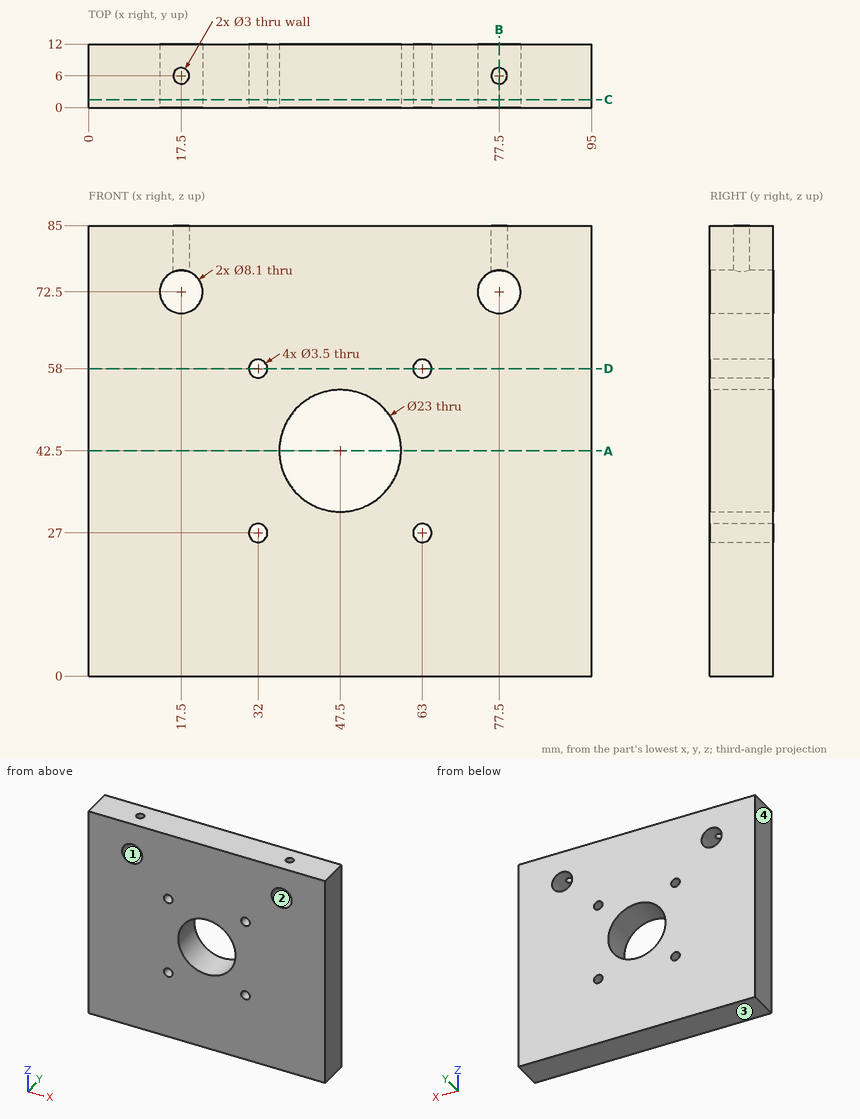
The drawing under review shows one solid part. Ordinate dimensions are in mm from its lowest x, y, z. Coordinates: 2 decimals unless noted, no trailing zeros. Write each loop counter-clockwise with the first axis right and the second up, starting at its lowest first coordinate (ties: lowest second). Pieces come first, ordered by that corner, then holes. Notation, with made-up numbers: (81.5, -1) -> (89.5, -1) arc R20 cw to (89.5, 14) -> close; hole circle Ø2 at (67, -26.75). An arc over 180 degrees is marked (long way). One line per item, written item: value. Start each with the question number.
Q1. Clearance check with a flat-ended pin moving along its axis: P1, Ø14, axis at x = 47.5, z = 42.5, coming from the +Y side. State where the tip first meets the part, or that it passes through.
Q2. Add section A-A, the plane z = 42.5. Give the boundary of the cut face in (x, y), then the cut area to 3 significant figures.
Q3. Add section D-D, the plane z = 58. Give the boundary of the cut face in (x, y).
Q4. Add section B-B, the plane x = 77.5. Give the boundary of the cut face in (y, z), then the cut area to 3 significant figures.
Q5. To check wall thickness, follow probe 1 along X at (y, z) = (6, 27); probe 2 along X at (y, z) = (7.5, 72.5); probe 3 along Z at (x, y) = (64, 7.5). State the ranges of each line that lie inside material, in increasing order.
Q6. Add section C-C, the plane y = 1.5. Give the boundary of the cut face in (x, z), then the cut area to 3 significant figures.
Q7. The part is to be moulded in two halves that separate along X. For the marked faces 1, 2, 3 and 4, say which applies: +X half, -X half, draft (parallel to the pull), parting line (faces both ways), or undercut.
Response:
1. P1: through
2. outline: (0, 0) -> (36, 0) -> (36, 12) -> (0, 12) -> close; (59, 0) -> (95, 0) -> (95, 12) -> (59, 12) -> close
2. area: 864 mm²
3. outline: (0, 0) -> (30.25, 0) -> (30.25, 12) -> (0, 12) -> close; (33.75, 0) -> (61.25, 0) -> (61.25, 12) -> (33.75, 12) -> close; (64.75, 0) -> (95, 0) -> (95, 12) -> (64.75, 12) -> close
4. outline: (0, 0) -> (12, 0) -> (12, 68.45) -> (0, 68.45) -> close; (0, 76.55) -> (4.5, 76.55) -> (4.5, 85) -> (0, 85) -> close; (7.5, 76.55) -> (12, 76.55) -> (12, 85) -> (7.5, 85) -> close
4. area: 897 mm²
5. probe 1: 0 to 30.25, 33.75 to 61.25, 64.75 to 95
5. probe 2: 0 to 13.45, 21.55 to 73.45, 81.55 to 95
5. probe 3: 0 to 25.56, 28.44 to 56.56, 59.44 to 85
6. outline: (0, 0) -> (95, 0) -> (95, 85) -> (0, 85) -> close; hole circle Ø8.1 at (17.5, 72.5); hole circle Ø3.5 at (32, 27); hole circle Ø3.5 at (32, 58); hole circle Ø23 at (47.5, 42.5); hole circle Ø3.5 at (63, 27); hole circle Ø3.5 at (63, 58); hole circle Ø8.1 at (77.5, 72.5)
6. area: 7,520 mm²
7. face 1: undercut
7. face 2: undercut
7. face 3: draft
7. face 4: -X half
